from build123d import *

# Parameters (mm, degrees)
SKETCH_1_W          = 20.5
SKETCH_1_H          = 30
EXTRUDE_1_DEPTH     = 30
FILLET_1_R          = 3
SKETCH_2_R          = 2.65
CUT_EXTRUDE_1_DEPTH = 84.693264365
SKETCH_3_R          = 2.65
CUT_EXTRUDE_2_DEPTH = 76.27491282
FILLET_2_R          = 3


with BuildPart() as part:
    # 草图1 → 凸台-拉伸1 (new body)
    # profile 1 of 2: a face of its own
    with BuildSketch(Plane.XY):
        Polygon((-13.25, -13.25), (-13.25, 10.25), (-13.25, 40.25), (-13.25, 63.75), (13.25, 63.75), (13.25, 40.25), (13.25, 10.25), (13.25, -13.25), align=None)
        Polygon((10.25, 40.25), (10.25, 60.75), (-10.25, 60.75), (-10.25, 40.25), (-10.25, 10.25), (-10.25, -10.25), (10.25, -10.25), (10.25, 10.25), align=None, mode=Mode.SUBTRACT)
    # profile 2 of 2: a face of its own
    with BuildSketch(Plane.XY):
        with Locations((0, 25.25)):
            Rectangle(SKETCH_1_W, SKETCH_1_H)
    extrude(amount=EXTRUDE_1_DEPTH)

    # 圆角1
    fillet_1_edges = [part.edges().sort_by_distance(p)[0] for p in [
        (-13.25, 63.75, 15),
        (13.25, 63.75, 15),
        (13.25, -13.25, 15),
        (-13.25, -13.25, 15),
    ]]
    fillet(fillet_1_edges, radius=FILLET_1_R)

    # 草图2 → 切除-拉伸1 (cut, through all)
    with BuildSketch(Plane(origin=(0, 63.75, 0), x_dir=(1, 0, 0), z_dir=(0, 1, 0))):
        with Locations(Location((0, -10, 0), (0, 0, 270))):
            Circle(SKETCH_2_R)
        with Locations(Location((0, -20, 0), (0, 0, 270))):
            Circle(SKETCH_2_R)
    extrude(amount=-CUT_EXTRUDE_1_DEPTH, mode=Mode.SUBTRACT)

    # 草图3 → 切除-拉伸2 (cut, through all)
    with BuildSketch(Plane(origin=(13.25, 0, 0), x_dir=(0, 0, -1), z_dir=(1, 0, 0))):
        with Locations((-10, 0)):
            Circle(SKETCH_3_R)
        with Locations((-20, 0)):
            Circle(SKETCH_3_R)
        with Locations(Location((-10, 50.5, 0), (0, 0, 180))):
            Circle(SKETCH_3_R)
        with Locations((-20, 50.5)):
            Circle(SKETCH_3_R)
    extrude(amount=-CUT_EXTRUDE_2_DEPTH, mode=Mode.SUBTRACT)

    # 圆角2
    fillet_2_edges = [part.edges().sort_by_distance(p)[0] for p in [
        (0, 40.25, 30),
        (0, 10.25, 0),
        (0, 40.25, 0),
        (0, 10.25, 30),
    ]]
    fillet(fillet_2_edges, radius=FILLET_2_R)


solid = part.part
Could you check a few things on this model? Use its own coordinates, in mm. A direction names the side the tool comes from. Coordinates: 2 decimals unless noted, no trailing zeros. Write each loop counter-clockwise with the first axis right and the second up, starting at its lowest first coordinate (ties: lowest second). Pieces come first, ordered by that corner, then holes. Notation, with made-up numbers: (26, 7.25) - (62, 7.25) arc R20 cw to (62, 42.25) - close; hole circle Ø9 at (-19, -25). An arc over 180 degrees is marked (long way). Put each result on its own line as item: value. Start each with the question number.
Q1. I want a section at B-B on y = 4.5. Write out the boundary of the cut face in (x, z), plus the area to 3 significant figures.
Q2. Please list where these lines run through material, in increasing order: L1, parallel to Y at x = 7.75, z = 4.25; L2, parallel to Z at x = 2.25, y = 37; L3, parallel to X at y = -3, z = 8.
Q3. I want a section at A-A on x = -7.75. Write out the boundary of the cut face in (y, z), plus the area to 3 significant figures.
Q4. I want a section at D-D on y = 38.5. Write out the boundary of the cut face in (x, z).
Q5. Thinking about a two-plate mould opening in X: for faces 6 (the flat face through (-13.25, 26, 15)), 7 (the cylindrical face through (11.771, 0.117, 12.647)), 8 (the flat face through (0, 60.75, 15)), which applies, pulls with the +X half, pulls with the -X half, needs draft (parallel to the pull), parting line crosses it, or undercut?
Q6. Which directions (+Z, -Z, +X, -X, +Y, -Y) give clear straight access to the entire face, cutting with the end or side of a thin tool? Please do faces 1 (the cylindrical face through (0.14, 39.35, 0.86)), 2 (the cylindrical face through (0.14, 11.15, 29.14)), 3 (the flat face through (0, -10.25, 15)), 4 (the cylindrical face through (0.117, 62.271, 7.353)), 5 (the cylindrical face through (-11.729, 52.734, 18.575)).
Q7. I want a section at C-C on z = 24. Write out the boundary of the cut face in (x, y), plus the area to 3 significant figures.
Q8. I'm going to push flat-ended pins straight in: P1, Ø3, axis at x = 0, z = 20, coming from the -Y side; P2, Ø1.5, axis at x = 2, y = 40.5, coming from the -Z side. Where does each tip first touch, or does it pass through?
Checks:
1. outline: (-13.25, 0) - (-10.25, 0) - (-10.25, 30) - (-13.25, 30) - close; (10.25, 0) - (13.25, 0) - (13.25, 30) - (10.25, 30) - close
1. area: 180 mm²
2. L1: -13.25 to -10.25, 10.25 to 40.25, 60.75 to 63.75
2. L2: 0 to 8.6, 11.4 to 18.6, 21.4 to 30
2. L3: -13.25 to -10.25, 10.25 to 13.25
3. outline: (-13.25, 0) - (-10.25, 0) - (-10.25, 30) - (-13.25, 30) - close; (10.25, 3) arc R3 ccw to (13.25, 0) - (37.25, 0) arc R3 ccw to (40.25, 3) - (40.25, 27) arc R3 ccw to (37.25, 30) - (13.25, 30) arc R3 ccw to (10.25, 27) - close; (60.75, 0) - (63.75, 0) - (63.75, 30) - (60.75, 30) - close
3. area: 1,070 mm²
4. outline: (-13.25, 0) - (-10.25, 0) - (-10.25, 0.27) - (10.25, 0.27) - (10.25, 0) - (13.25, 0) - (13.25, 30) - (10.25, 30) - (10.25, 29.73) - (-10.25, 29.73) - (-10.25, 30) - (-13.25, 30) - close; hole circle Ø5.3 at (0, 10); hole circle Ø5.3 at (0, 20)
5. face 6: pulls with the -X half
5. face 7: needs draft
5. face 8: undercut
6. face 1: -Z
6. face 2: +Z
6. face 3: +Z, -Z
6. face 4: +Y, -Y
6. face 5: +X, -X
7. outline: (-13.25, -10.25) arc R3 ccw to (-10.25, -13.25) - (10.25, -13.25) arc R3 ccw to (13.25, -10.25) - (13.25, 60.75) arc R3 ccw to (10.25, 63.75) - (-10.25, 63.75) arc R3 ccw to (-13.25, 60.75) - close; hole (-10.25, -10.25) - (10.25, -10.25) - (10.25, 10.25) - (-10.25, 10.25) - close; hole (-10.25, 40.25) - (10.25, 40.25) - (10.25, 60.75) - (-10.25, 60.75) - close
7. area: 1,190 mm²
8. P1: through
8. P2: z = 1.34
